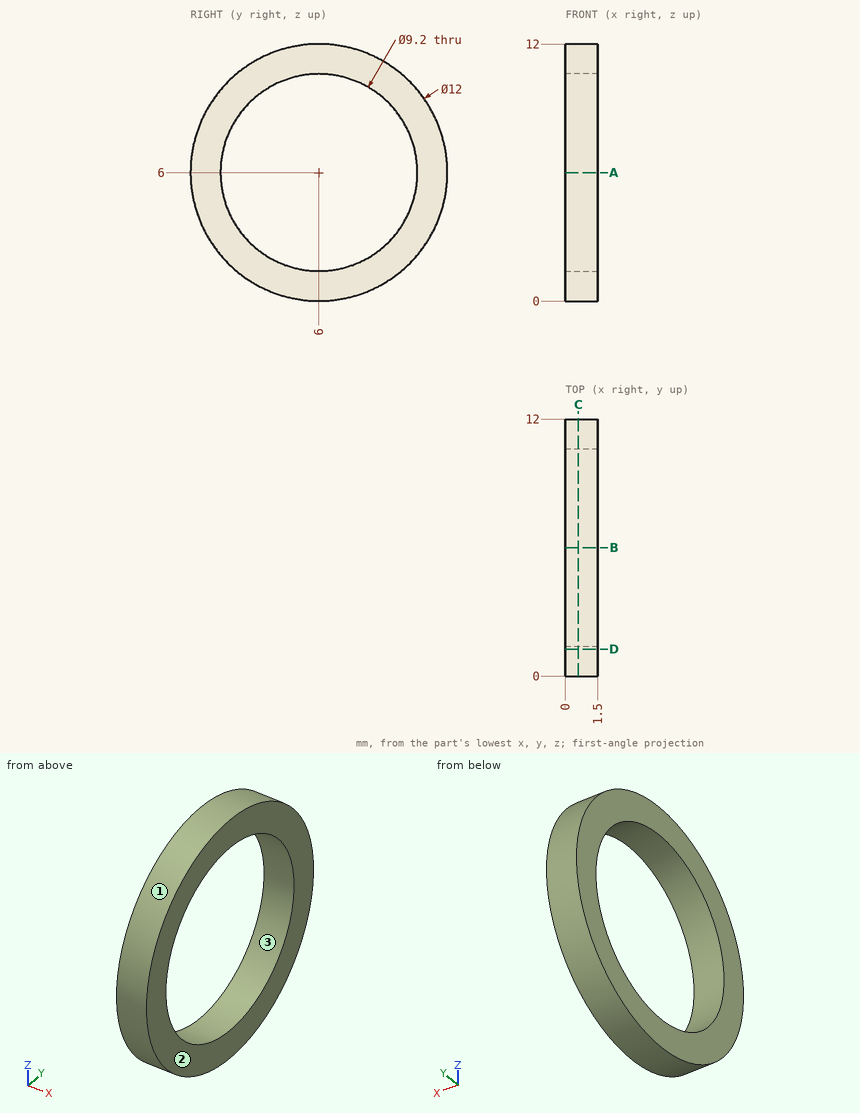
Study the drawing (mm; zero at the part's minimum x, y, z) and answer. Coordinates: 2 decimals unless noted, no trailing zeros. Loops run counter-clockwise (first coordinate to the right, second up) from the corner with the lowest first, then second, coordinate; pieces in that order, holes last. Notation, with made-up numbers: M 82,30.5 L 91,30.5 A32 cw 91,56.5 Z; hole C 33,73 d2. An arc over 180 degrees is marked long. Answer as a JSON object with one key per item and string values. Group by question number.
Item 1: Section A-A (z = 6) is taken. Write down the section's boundary in (x, y).
Item 2: Consider L1, parallel to Y at x = 1.1, z = 6; L2, parallel to Z at x = 0.65, y = 2.25; L3, parallel to Y at x = 0.45, z = 5.25. Determine where each line is inside the solid, lowest interval first.
Item 3: Section D-D (y = 1.25) is taken. Write down the section's boundary in (x, z), and give its area (3 significant figures).
Item 4: Determine the mould class of the marked faces 1, 2 and 3 for opening direction Z: +Z half, -Z half, draft (parallel to the pull), parting line (faces both ways), or undercut.
Item 5: Section C-C (x = 0.6) is taken. Write down the section's boundary in (y, z), and give its area (3 significant figures).
Solved:
{
 "1": {"outline": "M 0,0 L 1.5,0 L 1.5,1.4 L 0,1.4 Z; M 0,10.6 L 1.5,10.6 L 1.5,12 L 0,12 Z"},
 "2": {"L1": "y = 0 to 1.4, 10.6 to 12", "L2": "z = 1.32 to 3.34, 8.66 to 10.68", "L3": "y = 0.05 to 1.46, 10.54 to 11.95"},
 "3": {"outline": "M 0,2.33 L 1.5,2.33 L 1.5,9.67 L 0,9.67 Z", "area": "11.0 mm2"},
 "4": {"face 1": "parting line", "face 2": "draft", "face 3": "undercut"},
 "5": {"outline": "C 6,6 d12; hole C 6,6 d9.2", "area": "46.6 mm2"}
}
